Verification items for the finished model (mm, model axes). Face numbers are marked on the shaded views. A direction names the side the tool comes from. Coordinates: 2 decimals unless noted, no trailing zeros. Order: outer loops, then holes, each group sorted by start corner. A loop starts at its lowest first (then second) coordinate and runs counter-clockwise, first axis right, second up. Notation, with made-up numbers: (-8, -2.5) - (23, -2.5) arc R27 cw to (23, 35.5) - close; hole circle Ø11 at (83.25, 79). An arc over 180 degrees is marked (long way). Answer as CSV lines item,"result". Start each with the question number.
1. Set-up check for the marked faces 1 and 2: record each of +Z, -Z, +X, -X, +Y, -Y from which the full face is reachable in a straight line by a thin tool's end or side.
2. Section check B-B (y = -1.5). Record the cut outline in (x, z), and give its area (3 significant figures).
3. Section check C-C (y = 6.5). Record the cut outline in (x, z).
4. Section check D-D (x = -7.05). Record the cut outline in (y, z).
5. Go/stop test with flat-tipped pins: pin 1 (1 mm diameter, centred on x = -6.5, y = -5.5, fed in from +Z); pin 2 (4 mm diameter, centred on x = -8, z = 3.5, fed in from +Y); pin 3 (2.5 mm diameter, centred on y = -2, z = 2.5, fed in from -X). Record where each tip stops, or that it passes through.
6. Material ranges on L1, parallel to Y at x = -3.05, z = -2; L2, parallel to Z at x = -1.75, y = 5; L3, parallel to X at y = 6, z = 2.5, recorded low to high. Write a range as [from, to].
7. Mould release check, pull along Y, two halves, no side actions. Record for the marked faces 3, 4, 5 and 6: pulls with the +Y half, pulls with the -Y half, needs draft (parallel to the pull), parting line crosses it, or undercut.
8. Section check A-A (x = -4.25). Record the cut outline in (y, z).
from build123d import *

# Parameters (mm, degrees)
SKETCH_1_W          = 24.1
SKETCH_1_H          = 15
EXTRUDE_1_DEPTH     = 4
CUT_EXTRUDE_1_DEPTH = 15
EXTRUDE_2_DEPTH     = 0.9
SKETCH_4_R          = 1.5
CUT_EXTRUDE_2_DEPTH = 4
SKETCH_5_W          = 4
SKETCH_5_H          = 15
EXTRUDE_3_DEPTH     = 5


with BuildPart() as part:
    # 草图1 → 凸台-拉伸1 (new body)
    with BuildSketch(Plane.XY):
        Rectangle(SKETCH_1_W, SKETCH_1_H)
    extrude(amount=-EXTRUDE_1_DEPTH)

    # 草图2 → 切除-拉伸1 (cut)
    with BuildSketch(Plane.XZ.offset(7.5)):
        with BuildLine():
            Line((-8.05, 0), (-6.05, 0))
            ThreePointArc((-6.05, 0), (-7.05, -1), (-8.05, 0))
        make_face()
    extrude(amount=-CUT_EXTRUDE_1_DEPTH, mode=Mode.SUBTRACT)

    # 草图3 → 凸台-拉伸2 (add)
    with BuildSketch(Plane.XY):
        Polygon((-8.05, -6.462156705), (-8.05, -7.5), (-12.05, -7.5), (-12.05, -6.812111359), align=None)
    extrude(amount=EXTRUDE_2_DEPTH)

    # 草图4 → 切除-拉伸2 (cut)
    with BuildSketch(Plane.XY):
        with Locations((-3.05, -1.5)):
            Circle(SKETCH_4_R)
    extrude(amount=-CUT_EXTRUDE_2_DEPTH, mode=Mode.SUBTRACT)

    # 草图5 → 凸台-拉伸3 (add)
    with BuildSketch(Plane.XY):
        with Locations((10.05, 0)):
            Rectangle(SKETCH_5_W, SKETCH_5_H)
    extrude(amount=EXTRUDE_3_DEPTH)


solid = part.part
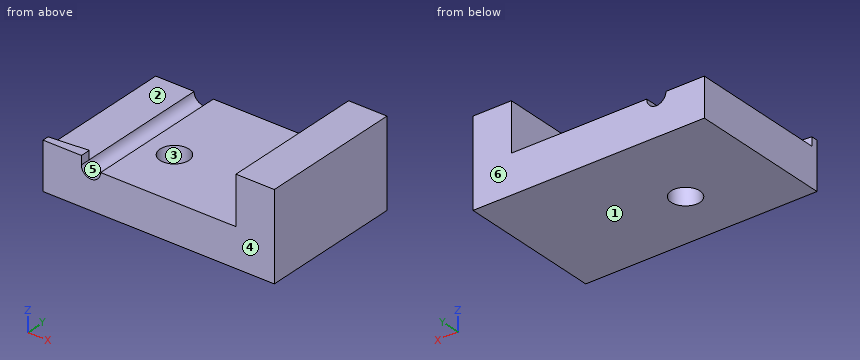
Evaluation:
1,face 1,"-Z, +X, -X, +Y, -Y"
1,face 2,"+Z, -X, +Y"
2,outline,"(-12.05, -4) - (-4.55, -4) - (-4.55, 0) - (-6.05, 0) arc R1 cw to (-8.05, 0) - (-12.05, 0) - close; (-1.55, -4) - (12.05, -4) - (12.05, 5) - (8.05, 5) - (8.05, 0) - (-1.55, 0) - close"
2,area,"103 mm²"
3,outline,"(-12.05, -4) - (12.05, -4) - (12.05, 5) - (8.05, 5) - (8.05, 0) - (-6.05, 0) arc R1 cw to (-8.05, 0) - (-12.05, 0) - close"
4,outline,"(-7.5, -4) - (7.5, -4) - (7.5, -1) - (-7.5, -1) - close"
5,pin 1,"stops at z = 0"
5,pin 2,"passes through"
5,pin 3,"stops at x = 8.05"
6,L1,"y = [-7.5, -3], [0, 7.5]"
6,L2,"z = [-4, 0]"
6,L3,"x = [8.05, 12.05]"
7,face 3,"undercut"
7,face 4,"pulls with the -Y half"
7,face 5,"needs draft"
7,face 6,"pulls with the +Y half"
8,outline,"(-7.5, -4) - (-2.4, -4) - (-2.4, 0) - (-7.5, 0) - close; (-0.6, -4) - (7.5, -4) - (7.5, 0) - (-0.6, 0) - close"
